from build123d import *

# Parameters (mm, degrees)
SKETCH_R     = 5
SKETCH_R_2   = 3
PAD_DEPTH    = 20
SKETCH002_R  = 2
PAD001_DEPTH = 5
SKETCH003_R  = 3
POCKET_DEPTH = 20.001
FILLET_R     = 1


with BuildPart() as body:
    # Sketch → Pad (new body)
    with BuildSketch(Plane.XY):
        Circle(SKETCH_R)
        Circle(SKETCH_R_2, mode=Mode.SUBTRACT)
    extrude(amount=PAD_DEPTH)


with BuildPart() as body002:
    # Sketch002 → Pad001 (new body, symmetric)
    with BuildSketch(Plane.XZ):
        Polygon((9.975506, 17.427483), (0, 20), (0, 0), (9.975506, 2.572517), align=None)
        with Locations((7, 10)):
            Circle(SKETCH002_R, mode=Mode.SUBTRACT)
    extrude(amount=PAD001_DEPTH, both=True)

    # Boolean: union Body
    add(body.part)

    # Sketch003 (on Face11 of Boolean) → Pocket (cut, through all)
    with BuildSketch(Plane(origin=(0, 0, 0), x_dir=(1, 0, 0), z_dir=(0, 0, -1))):
        Circle(SKETCH003_R)
    extrude(amount=-POCKET_DEPTH, mode=Mode.SUBTRACT)

    # Fillet
    fillet_edges = [body002.edges().sort_by_distance(p)[0] for p in [
        (9.975506, -5, 10),
        (9.975506, 5, 10),
    ]]
    fillet(fillet_edges, radius=FILLET_R)


solid = body002.part
Geometry check sheet. Reference: the model listing, model coordinates, mm. A direction names the side the tool comes from. Coordinates: 2 decimals unless noted, no trailing zeros. Loops run counter-clockwise (first coordinate to the right, second up) from the corner with the lowest first, then second, coordinate; pieces in that order, holes last. Notation, with made-up numbers: (59, 18) - (92, 18) arc R33 ccw to (92, 52) - close; hole circle Ø5 at (89, 85.5). An arc over 180 degrees is marked (long way). Use one line per item in the form item = value. Start each with the question number.
Item 1: Gauge pin test, flat ends, axial feed: pin 1 (3 mm diameter, centred on x = 7, z = 10, fed in from +Y); pin 2 (4 mm diameter, centred on x = -2.5, z = 12.5, fed in from +Y); pin 3 (6 mm diameter, centred on x = 7.5, y = -1, fed in from +Z). Record the tip position at first contact, or that the pin passes through.
Item 2: Thickness scan on probe 1 along X at (y, z) = (1.75, 10); probe 2 along X at (y, z) = (-1, 10); probe 3 along Y at (x, z) = (-0.75, 6.5). Record the ranges inside material, lowest first.
Item 3: Mould release check, pull along Z, two halves, no side actions. Record for faces 4 (the face through (-0.1, -3.3, 0)), 5 (the face through (9.69, 4.7, 14.05)), 6 (the face through (5.526, 0.07, 11.352)): +Z half, -Z half, draft (parallel to the pull), parting line (faces both ways), or undercut.
Item 4: Section check D-D, the plane y = -2.25. Enter the section's corners in (x, z).
Item 5: Tool access check on faces 1 (the face through (5, 0, 19)), 2 (the face through (4, 5, 10)), 3 (the face through (5, -0.1, 0.5)). Record the directions out of +Z, -Z, +X, -X, +Y, -Y that give a thin tool (end or side, any length) a straight path to the whole face; none if there is none.
Item 6: Section check A-A, the plane y = 1.75. Enter the section's corners in (x, z).
Item 7: Section check B-B, the plane z = 16.75. Enter the section's corners in (x, y).
Computed:
q1.pin_1 = through
q1.pin_2 = 4.97
q1.pin_3 = 20
q2.probe_1 = -4.68 to -2.44, 2.44 to 5, 9 to 9.98
q2.probe_2 = -4.9 to -2.83, 2.83 to 5, 9 to 9.98
q2.probe_3 = -4.94 to -2.9, 2.9 to 4.94
q3.face_4 = -Z half
q3.face_5 = draft
q3.face_6 = undercut
q4.outline = (-4.47, 0) - (-1.98, 0) - (-1.98, 20) - (-4.47, 20) - close; (1.98, 0) - (4.47, 0) - (4.47, 1.15) - (9.98, 2.57) - (9.98, 17.43) - (4.47, 18.85) - (4.47, 20) - (1.98, 20) - close; hole circle Ø4 at (7, 10)
q5.face_1 = +Z, +X
q5.face_2 = +Z, -Z, +X, -X, +Y
q5.face_3 = -Z, +X
q6.outline = (-4.68, 0) - (-2.44, 0) - (-2.44, 20) - (-4.68, 20) - close; (2.44, 0) - (4.68, 0) - (4.68, 1.21) - (9.98, 2.57) - (9.98, 17.43) - (4.68, 18.79) - (4.68, 20) - (2.44, 20) - close; hole circle Ø4 at (7, 10)
q7.outline = (0, -5) - (8.98, -5) arc R1 ccw to (9.98, -4) - (9.98, 4) arc R1 ccw to (8.98, 5) - (0, 5) arc R5 ccw to start; hole circle Ø6 at (0, 0)
